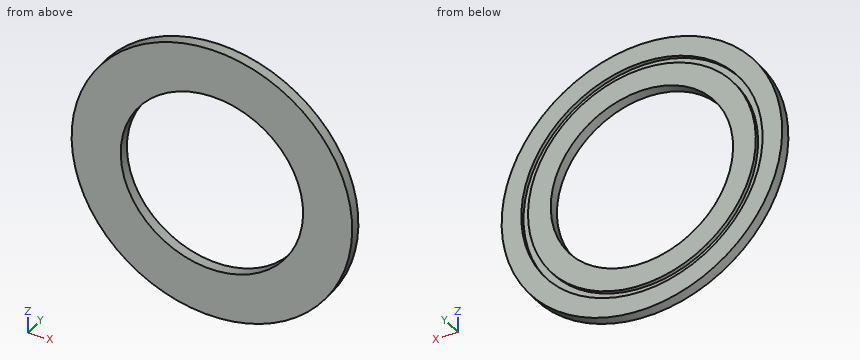
```python
from build123d import *

# Parameters (mm, degrees)
SKETCH1_R           = 250
SKETCH1_R_2         = 162.5
BOSS_EXTRUDE1_DEPTH = 19
SKETCH2_R           = 215
SKETCH2_R_2         = 203
CUT_EXTRUDE1_DEPTH  = 7


with BuildPart() as part:
    # Sketch1 → Boss-Extrude1 (new body)
    with BuildSketch(Plane(origin=(0, 0, 0), x_dir=(1, 0, 0), z_dir=(0, 1, 0))):
        with Locations(Location((0, 0, 0), (0, 0, 270))):
            Circle(SKETCH1_R)
        with Locations(Location((0, 0, 0), (0, 0, 270))):
            Circle(SKETCH1_R_2, mode=Mode.SUBTRACT)
    extrude(amount=BOSS_EXTRUDE1_DEPTH)

    # Sketch2 → Cut-Extrude1 (cut)
    with BuildSketch(Plane(origin=(0, 19, 0), x_dir=(1, 0, 0), z_dir=(0, 1, 0))):
        with Locations(Location((0, 0, 0), (0, 0, 270))):
            Circle(SKETCH2_R)
        with Locations(Location((0, 0, 0), (0, 0, 270))):
            Circle(SKETCH2_R_2, mode=Mode.SUBTRACT)
    extrude(amount=-CUT_EXTRUDE1_DEPTH, mode=Mode.SUBTRACT)


solid = part.part
```
Here's how the part is built. I have some questions about the finished solid (model axes, mm). Give positions to 0.01 mm unless a question says otherwise; leave off trailing zeros. Loops run counter-clockwise (first coordinate to the right, second up) from the corner with the lowest first, then second, coordinate; pieces in that order, holes last. Notation, with made-up numbers: M 36.5,23 L 88.5,23 A19 ccw 88.5,33 Z; hole C -40,60.25 d6. An arc over 180 degrees is marked long. Put each result on its own line as item: value. Start each with the question number.
(1) I need wall thicknesses on line 1 along X through (y, z) = (14, 0); line 2 along X through (y, z) = (13, 92); line 3 along X through (y, z) = (5.5, 0). Which ranges of each line are inside material? Lowest first, please. Write a range as [from, to].
(2) I want a section at A-A on z = 0. Please give me the cut outline in (x, y).
(3) I want a section at D-D on x = -189.5. Please give me the cut outline in (y, z).
(4) Will these pins go through, and if not, where does the flat tip stop? pin 1 Ø4 at (y, z) = (10.5, -52.5) entering from +X; pin 2 Ø1.5 at (y, z) = (16, -63) entering from -X; pin 3 Ø5 at (x, y) = (148, 6.5) entering from +Z.
(5) I want a section at C-C on y = 7. Please give me the cut outline in (x, z).
(6) I want a section at B-B on x = 0. Please give me the cut outline in (y, z).
Answer block:
1. line 1: [-250, -215], [-203, -162.5], [162.5, 203], [215, 250]
1. line 2: [-232.46, -194.32], [-180.96, -133.95], [133.95, 180.96], [194.32, 232.46]
1. line 3: [-250, -162.5], [162.5, 250]
2. outline: M -250,0 L -162.5,0 L -162.5,19 L -203,19 L -203,12 L -215,12 L -215,19 L -250,19 Z; M 162.5,0 L 250,0 L 250,19 L 215,19 L 215,12 L 203,12 L 203,19 L 162.5,19 Z
3. outline: M 0,-163.06 L 19,-163.06 L 19,-101.56 L 12,-101.56 L 12,-72.79 L 19,-72.79 L 19,72.79 L 12,72.79 L 12,101.56 L 19,101.56 L 19,163.06 L 0,163.06 Z
4. pin 1: x = 244.85
4. pin 2: x = -242.13
4. pin 3: z = 203.3
5. outline: C 0,0 d500; hole C 0,0 d325
6. outline: M 0,-250 L 19,-250 L 19,-215 L 12,-215 L 12,-203 L 19,-203 L 19,-162.5 L 0,-162.5 Z; M 0,162.5 L 19,162.5 L 19,203 L 12,203 L 12,215 L 19,215 L 19,250 L 0,250 Z
